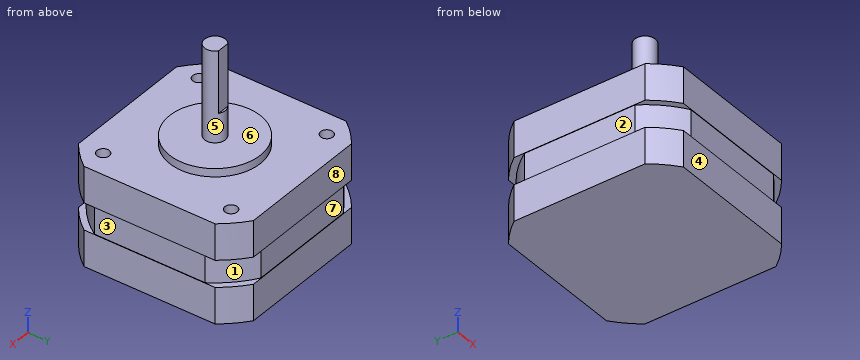
from build123d import *

# Parameters (mm, degrees)
SKETCH1_R                       = 2.5
BOSS_EXTRUDE1_DEPTH             = 24
SKETCH2_R                       = 11
BOSS_EXTRUDE2_DEPTH             = 2
SKETCH3_W                       = 42.418
SKETCH3_H                       = 42.418
BOSS_EXTRUDE3_DEPTH             = 24
CUT_EXTRUDE1_DEPTH              = 49
M3X0_5_TAPPED_HOLE1_D           = 2.5
M3X0_5_TAPPED_HOLE1_DEPTH       = 7.5
M3X0_5_TAPPED_HOLE1_CBORE_D     = 3
M3X0_5_TAPPED_HOLE1_CBORE_DEPTH = 6
M3X0_5_TAPPED_HOLE1_TIP         = 0.751075774
CUT_EXTRUDE2_DEPTH              = 15
CUT_EXTRUDE3_DEPTH              = 3.25
CUT_EXTRUDE3_DEPTH_BACK         = 3.25


with BuildPart() as part:
    # Sketch1 → Boss-Extrude1 (new body)
    with BuildSketch(Plane.XY):
        Circle(SKETCH1_R)
    extrude(amount=BOSS_EXTRUDE1_DEPTH)

    # Sketch2 → Boss-Extrude2 (add)
    with BuildSketch(Plane(origin=(0, 0, 0), x_dir=(-1, 0, 0), z_dir=(0, 0, -1))):
        Circle(SKETCH2_R)
    extrude(amount=-BOSS_EXTRUDE2_DEPTH)

    # Sketch3 → Boss-Extrude3 (add)
    with BuildSketch(Plane(origin=(0, 0, 0), x_dir=(-1, 0, 0), z_dir=(0, 0, -1))):
        Rectangle(SKETCH3_W, SKETCH3_H)
    extrude(amount=BOSS_EXTRUDE3_DEPTH)

    # Sketch4 → Cut-Extrude1 (cut, through all)
    with BuildSketch(Plane(origin=(0, 0, -24), x_dir=(-1, 0, 0), z_dir=(0, 0, -1))):
        with BuildLine():
            Line((-21.209, -15.887992919), (-21.209, -21.209))
            Line((-21.209, -21.209), (-15.887992919, -21.209))
            ThreePointArc((-15.887992919, -21.209), (-18.738329701, -18.738329701), (-21.209, -15.887992919))
        make_face()
        with BuildLine():
            Line((15.887992919, -21.209), (21.209, -21.209))
            Line((21.209, -21.209), (21.209, -15.887992919))
            ThreePointArc((21.209, -15.887992919), (18.738329701, -18.738329701), (15.887992919, -21.209))
        make_face()
        with BuildLine():
            Line((21.209, 15.887992919), (21.209, 21.209))
            Line((21.209, 21.209), (15.887992919, 21.209))
            ThreePointArc((15.887992919, 21.209), (18.738329701, 18.738329701), (21.209, 15.887992919))
        make_face()
        with BuildLine():
            Line((-15.887992919, 21.209), (-21.209, 21.209))
            Line((-21.209, 21.209), (-21.209, 15.887992919))
            ThreePointArc((-21.209, 15.887992919), (-18.738329701, 18.738329701), (-15.887992919, 21.209))
        make_face()
    extrude(amount=-CUT_EXTRUDE1_DEPTH, mode=Mode.SUBTRACT)

    # M3x0.5 Tapped Hole1
    with Locations(Plane.XY):
        with Locations((-15.5, 15.5), (-15.5, -15.5), (15.5, -15.5), (15.5, 15.5)):
            CounterBoreHole(M3X0_5_TAPPED_HOLE1_D / 2, M3X0_5_TAPPED_HOLE1_CBORE_D / 2, M3X0_5_TAPPED_HOLE1_CBORE_DEPTH, depth=M3X0_5_TAPPED_HOLE1_DEPTH)
            with Locations((0, 0, -(M3X0_5_TAPPED_HOLE1_DEPTH + M3X0_5_TAPPED_HOLE1_TIP / 2))):  # 118° drill point
                Cone(0, M3X0_5_TAPPED_HOLE1_D / 2, M3X0_5_TAPPED_HOLE1_TIP, mode=Mode.SUBTRACT)

    # Sketch7 → Cut-Extrude2 (cut)
    with BuildSketch(Plane.XY.offset(24)):
        with BuildLine():
            Line((-1.5, 2), (1.5, 2))
            ThreePointArc((1.5, 2), (0, 2.5), (-1.5, 2))
        make_face()
    extrude(amount=-CUT_EXTRUDE2_DEPTH, mode=Mode.SUBTRACT)

    # Sketch8 → Cut-Extrude3 (cut, two sides)
    with BuildSketch(Plane.XY.offset(-12)) as cut_extrude3_sk:
        with BuildLine():
            Line((15.887992919, 21.209), (-15.887992919, 21.209))
            ThreePointArc((-15.887992919, 21.209), (-18.738329701, 18.738329701), (-21.209, 15.887992919))
            Line((-21.209, 15.887992919), (-21.209, -15.887992919))
            ThreePointArc((-21.209, -15.887992919), (-18.738329701, -18.738329701), (-15.887992919, -21.209))
            Line((-15.887992919, -21.209), (15.887992919, -21.209))
            ThreePointArc((15.887992919, -21.209), (18.738329701, -18.738329701), (21.209, -15.887992919))
            Line((21.209, -15.887992919), (21.209, 15.887992919))
            ThreePointArc((21.209, 15.887992919), (18.738329701, 18.738329701), (15.887992919, 21.209))
        make_face()
        with BuildLine():
            Line((-13.394406258, 21.109), (13.394406258, 21.109))
            ThreePointArc((13.394406258, 21.109), (17.67766953, 17.67766953), (21.109, 13.394406258))
            Line((21.109, 13.394406258), (21.109, -13.394406258))
            ThreePointArc((21.109, -13.394406258), (17.67766953, -17.67766953), (13.394406258, -21.109))
            Line((13.394406258, -21.109), (-13.394406258, -21.109))
            ThreePointArc((-13.394406258, -21.109), (-17.67766953, -17.67766953), (-21.109, -13.394406258))
            Line((-21.109, -13.394406258), (-21.109, 13.394406258))
            ThreePointArc((-21.109, 13.394406258), (-17.67766953, 17.67766953), (-13.394406258, 21.109))
        make_face(mode=Mode.SUBTRACT)
    extrude(amount=CUT_EXTRUDE3_DEPTH, mode=Mode.SUBTRACT)
    extrude(cut_extrude3_sk.sketch, amount=-CUT_EXTRUDE3_DEPTH_BACK, mode=Mode.SUBTRACT)


solid = part.part
The model under review builds one solid part; all positions refer to its coordinate system, in mm. Face numbers are marked on the shaded views. A direction names the side the tool comes from. Give positions to 0.01 mm unless a question says otherwise; leave off trailing zeros. Order: outer loops, then holes, each group sorted by start corner. A loop starts at its lowest first (then second) coordinate and runs counter-clockwise, first axis right, second up. Notation, with made-up numbers: M -22.75,39.25 L 1.25,39.25 A9 ccw 1.25,46.25 Z; hole C -11,22 d10. An arc over 180 degrees is marked long. Answer in a Markdown table with one row per item. Add a question column.
1. Mouldability with a two-part tool opening along Z and no side actions: class the marked faces 6, 7 and 8 as released by +Z, released by -Z, zero draft, split by the parting line, or undercut.
2. To check wall thickness, follow line 1 along Y through (x, z) = (-15.5, -6.75); line 2 along Y through (x, z) = (-15.5, -2.6). State the ranges of each line that lie inside material, in increasing order.
3. Add section A-A on x = 0. State the section outline as (y, z) points, plus the area to 3 significant figures.
4. Add section C-C on z = 17.5. State the section outline as (x, y) points, plus the area to 3 significant figures.
5. For pin 1 Ø3.5 at (x, y) = (-15, 16) entering from +Z; pin 2 Ø8 at (x, z) = (-12, -13) entering from -Y; pin 3 Ø3 at (x, z) = (-0.5, -13.5) entering from +Y; pin 4 Ø10 at (x, y) = (-4, 13.5) entering from +Z, all flat-tipped, find the tip position at first contact; note any pin that passes through.
6. Machinability: for the marked faces 1, 2, 3, 4 and 5, which of the approach directions +Z, -Z, +X, -X, +Y, -Y give a long, thin tool a straight path to every point of the face, cutting with its end or side? Answer none if there is none.
7. Add section B-B on y = 0. State the section outline as (x, z) points.
8. Add section D-D on y = -8. State the section outline as (x, z) points.
The answers:
| question | item | result |
|---|---|---|
| 1 | face 6 | released by +Z |
| 1 | face 7 | undercut |
| 1 | face 8 | zero draft |
| 2 | line 1 | -21.21 to -16.75, -14.25 to 14.25, 16.75 to 21.21 |
| 2 | line 2 | -21.21 to -17, -14 to 14, 17 to 21.21 |
| 3 | outline | M -21.21,-24 L 21.21,-24 L 21.21,-15.25 L 21.11,-15.25 L 21.11,-8.75 L 21.21,-8.75 L 21.21,0 L 11,0 L 11,2 L 2.5,2 L 2.5,9 L 2,9 L 2,24 L -2.5,24 L -2.5,2 L -11,2 L -11,0 L -21.21,0 L -21.21,-8.75 L -21.11,-8.75 L -21.11,-15.25 L -21.21,-15.25 Z |
| 3 | area | 1,160 mm2 |
| 4 | outline | M -1.5,2 A2.5 ccw long 1.5,2 Z |
| 4 | area | 18.6 mm2 |
| 5 | pin 1 | z = 0 |
| 5 | pin 2 | y = -21.21 |
| 5 | pin 3 | y = 21.11 |
| 5 | pin 4 | z = 2 |
| 6 | face 1 | +X, +Y |
| 6 | face 2 | -X, +Y, -Y |
| 6 | face 3 | +X, +Y, -Y |
| 6 | face 4 | +Z, -Z, +X, -X, -Y |
| 6 | face 5 | +Z |
| 7 | outline | M -21.21,-24 L 21.21,-24 L 21.21,-15.25 L 21.11,-15.25 L 21.11,-8.75 L 21.21,-8.75 L 21.21,0 L 11,0 L 11,2 L 2.5,2 L 2.5,24 L -2.5,24 L -2.5,2 L -11,2 L -11,0 L -21.21,0 L -21.21,-8.75 L -21.11,-8.75 L -21.11,-15.25 L -21.21,-15.25 Z |
| 8 | outline | M -21.21,-24 L 21.21,-24 L 21.21,-15.25 L 21.11,-15.25 L 21.11,-8.75 L 21.21,-8.75 L 21.21,0 L 7.55,0 L 7.55,2 L -7.55,2 L -7.55,0 L -21.21,0 L -21.21,-8.75 L -21.11,-8.75 L -21.11,-15.25 L -21.21,-15.25 Z |
